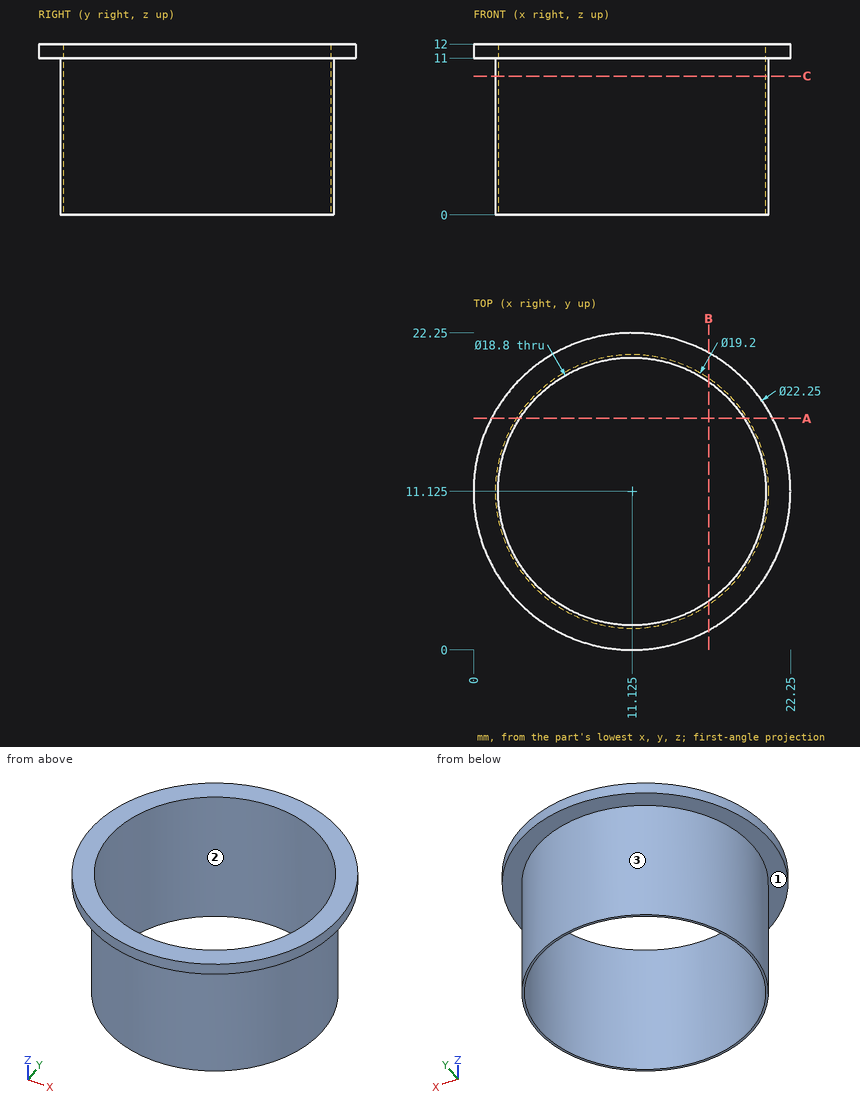
Check sheet for the drawn part. Datum: minimum x, y, z corner. Units: mm. Round coordinates to 2 decimals unless told otherwise and drop trailing zeros. Order: outer loops, then holes, each group sorted by start corner. A loop starts at its lowest first (then second) coordinate and runs counter-clockwise, first axis right, second up. Notation, with made-up numbers: (5.25, 88.5) - (61.25, 88.5) arc R22 cw to (61.25, 115.5) - close; hole circle Ø9 at (-8, 65.25). An arc over 180 degrees is marked (long way). Use a Markdown table: item, result. Add a question column.
(1) Sectioned sample at B-B, the plane x = 16.5. Enter the section's corners in (y, z), and give its area (3 significant figures).
(2) Sectioned sample at C-C, the plane z = 9.75. Enter the section's corners in (x, y) (3 decimals).
(3) Sectioned sample at A-A, the plane y = 16.25. Enter the section's corners in (x, z) (3 decimals).
(4) Release check for a two-part mould opening along Y. For the marked faces 1, 2 and 3 record: pulls with the +Y half, pulls with the -Y half, needs draft (parallel to the pull), parting line crosses it, or undercut.
(5) Depth check by flat-ended pin: pin 1 (2 mm diameter, centred on y = 2.5, z = 8.5, fed in from +X); pin 2 (3 mm diameter, centred on x = 9.5, z = 8.5, fed in from +Y); pin 3 (2 mm diameter, centred on y = 11, z = 6, fed in from +X) (3 decimals). Enter the tip coordinate at first touch or a pass-through.
(6) Material ranges on line 1 along Z through (x, y) = (6, 19.5); line 2 along X through (y, z) = (11.5, 10); line 3 along Y through (x, z) = (19, 11.25), recorded low to high. Write a range as [from, to].
Answers below:
| question | item | result |
|---|---|---|
| 1 | outline | (1.38, 11) - (3.17, 11) - (3.17, 0) - (3.41, 0) - (3.41, 12) - (1.38, 12) - close; (18.84, 0) - (19.08, 0) - (19.08, 11) - (20.87, 11) - (20.87, 12) - (18.84, 12) - close |
| 1 | area | 9.39 mm² |
| 2 | outline | circle Ø19.2 at (11.125, 11.125); hole circle Ø18.8 at (11.125, 11.125) |
| 3 | outline | (1.251, 11) - (3.007, 11) - (3.007, 0) - (3.245, 0) - (3.245, 12) - (1.251, 12) - close; (19.005, 0) - (19.243, 0) - (19.243, 11) - (20.999, 11) - (20.999, 12) - (19.005, 12) - close |
| 4 | face 1 | needs draft |
| 4 | face 2 | undercut |
| 4 | face 3 | parting line crosses it |
| 5 | pin 1 | x = 16.96 |
| 5 | pin 2 | y = 20.72 |
| 5 | pin 3 | x = 20.725 |
| 6 | line 1 | [11, 12] |
| 6 | line 2 | [1.53, 1.73], [20.52, 20.72] |
| 6 | line 3 | [3.27, 5.99], [16.26, 18.98] |
